Input: part model. Units: mm. Frame: model coordinates. Face numbers are marked on the shaded views. A direction names the side the tool comes from. Round coordinates to 2 decimals unless told otherwise and drop trailing zeros. Order: outer loops, then holes, each group sorted by start corner. A loop starts at its lowest first (then second) coordinate and runs counter-clockwise, first axis right, second up. Notation, with made-up numbers: (11, 64.25) - (62, 64.25) arc R23 cw to (62, 87.25) - close; hole circle Ø11 at (-37.5, 18.25). An arc over 180 degrees is marked (long way). One line per item, written item: value. Start each with the question number.
from build123d import *

# Parameters (mm, degrees)
ESQUISSE1_R        = 2.5
BOSS_EXTRU_2_DEPTH = 2
ESQUISSE2_R        = 2.5
ESQUISSE2_W        = 15
ESQUISSE2_H        = 2
BOSS_EXTRU_3_DEPTH = 2
CONG_1_R           = 2
CONG_2_R           = 2
CONG_4_R           = 1


with BuildPart() as part:
    # Esquisse1 → Boss.-Extru.2 (new body)
    with BuildSketch(Plane(origin=(0, 0, 0), x_dir=(1, 0, 0), z_dir=(0, 1, 0))):
        with BuildLine():
            ThreePointArc((-7.5, 0), (0, -7.5), (7.5, 0))
            Line((7.5, 0), (7.5, 32.5))
            Line((7.5, 32.5), (-7.5, 32.5))
            Line((-7.5, 32.5), (-7.5, 0))
        make_face()
        with Locations(Location((0, -2, 0), (0, 0, 270))):
            Circle(ESQUISSE1_R, mode=Mode.SUBTRACT)
        with Locations(Location((0, 18, 0), (0, 0, 270))):
            Circle(ESQUISSE1_R, mode=Mode.SUBTRACT)
    extrude(amount=BOSS_EXTRU_2_DEPTH)

    # Esquisse2 → Boss.-Extru.3 (add)
    # profile 1 of 2: a face of its own
    with BuildSketch(Plane(origin=(0, 0, -32.5), x_dir=(-1, 0, 0), z_dir=(0, 0, -1))):
        with BuildLine():
            Line((-7.5, 32.5), (-7.5, 2))
            Line((-7.5, 2), (7.5, 2))
            Line((7.5, 2), (7.5, 32.5))
            ThreePointArc((7.5, 32.5), (5.303300859, 37.803300859), (0, 40))
            ThreePointArc((0, 40), (-5.303300859, 37.803300859), (-7.5, 32.5))
        make_face()
        with Locations((0, 14.5)):
            Circle(ESQUISSE2_R, mode=Mode.SUBTRACT)
        with Locations((0, 34.5)):
            Circle(ESQUISSE2_R, mode=Mode.SUBTRACT)
    # profile 2 of 2: a face of its own
    with BuildSketch(Plane(origin=(0, 0, -32.5), x_dir=(-1, 0, 0), z_dir=(0, 0, -1))):
        with Locations((0, 1)):
            Rectangle(ESQUISSE2_W, ESQUISSE2_H)
    extrude(amount=-BOSS_EXTRU_3_DEPTH)

    # Congé1
    cong_1_edges = [part.edges().sort_by_distance(p)[0] for p in [
        (0, 0, -32.5),
    ]]
    fillet(cong_1_edges, radius=CONG_1_R)

    # Congé2
    cong_2_edges = [part.edges().sort_by_distance(p)[0] for p in [
        (0, 2, -30.5),
    ]]
    fillet(cong_2_edges, radius=CONG_2_R)

    # Congé4
    cong_4_edges = [part.edges().sort_by_distance(p)[0] for p in [
        (0, 2, 7.5),
        (7.5, 2, -14.25),
        (0, 40, -30.5),
        (-7.5, 2, -14.25),
        (7.5, 18.25, -30.5),
        (-7.5, 18.25, -30.5),
        (-7.5, 2.585786438, -29.914213562),
        (7.5, 2.585786438, -29.914213562),
    ]]
    fillet(cong_4_edges, radius=CONG_4_R)


solid = part.part
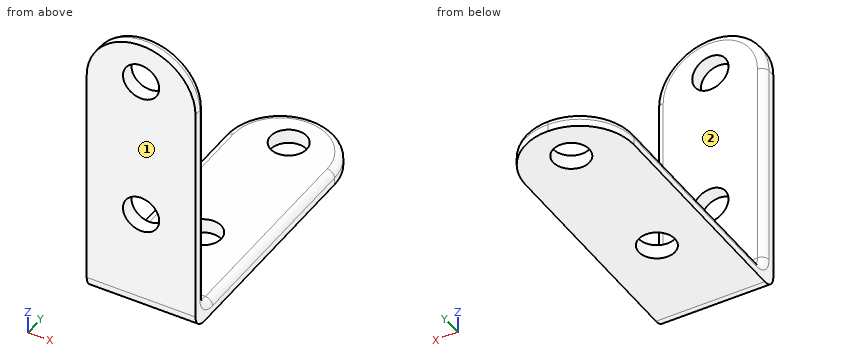
1. Pin query (flat end, axial travel): pin 1 (6.5 mm diameter, centred on x = 0, z = 2, fed in from +Y); pin 2 (1 mm diameter, centred on x = 4, y = 12.5, fed in from +Z). Return the tip coordinate at first contact, or that it passes through.
2. Section D-D (x = 1). State how many separate pieces and enclosed holes the cut face has, then the cut area to 3 significant figures.
3. Section A-A (y = 14.5). Return the cut outline in (x, z).
4. Section B-B (z = -7.5). Return the cut outline in (x, y).
5. Set-up query: the marked faces 1 and 2. Return all of +Z, -Z, +X, -X, +Y, -Y with unobstructed straight access to the full face (end or side cutting, diameter ignored); none if empty.
6. Line query: line 1 (X direction, y = 1, z = -18); line 2 (Y direction, x = 0, z = -31.7); line 3 (Y direction, x = -5.75, z = -9). Output: solid intervals per line, ascending. Write a range as from..to.
7. Section C-C (y = 9). Return the cut outline in (x, z).
Solved:
1. pin 1: stops at y = 2
1. pin 2: stops at z = -30.5
2. separate pieces: 5
2. enclosed holes: 0
2. area: 119 mm²
3. outline: (-7.5, -32.5) - (-2.5, -32.5) - (-2.5, -30.5) - (-6.5, -30.5) arc R1 ccw to (-7.5, -31.5) - close; (2.5, -32.5) - (7.5, -32.5) - (7.5, -31.5) arc R1 ccw to (6.5, -30.5) - (2.5, -30.5) - close
4. outline: (-7.5, 0) - (7.5, 0) - (7.5, 1) arc R1 ccw to (6.5, 2) - (-6.5, 2) arc R1 ccw to (-7.5, 1) - close
5. face 1: +Z, -Z, +X, -X, -Y
5. face 2: +Z, +X, -X, +Y
6. line 1: x = -7.5..-2.5, 2.5..7.5
6. line 2: y = 0.4..12, 17..32, 37..40
6. line 3: y = 0..2
7. outline: (-7.5, -32.5) - (7.5, -32.5) - (7.5, -31.5) arc R1 ccw to (6.5, -30.5) - (-6.5, -30.5) arc R1 ccw to (-7.5, -31.5) - close
